Design review of the part shown in the three views and the two pictorial views. Dimensions are in mm from the part's minimum x, y and z. A direction names the side the tool comes from. Round coordinates to 2 decimals unless told otherwise and drop trailing zeros. Loops run counter-clockwise (first coordinate to the right, second up) from the corner with the lowest first, then second, coordinate; pieces in that order, holes last.
1. To check wall thickness, follow line 1 along Y through (x, z) = (2.6, 7); line 2 along Z through (x, y) = (3.45, 1.5); line 3 along Z through (x, y) = (2.35, 2.5). State the ranges of each line that lie inside material, in increasing order.
2. Tool access review of the marked faces 1 and 2: name each direction out of +Z, -Z, +X, -X, +Y, -Y from which nothing blocks a thin tool from reaching the whole face with its end or side.
3. Clearance check with a flat-ended pin moving along its axis: pin 1 Ø0.6 at (x, y) = (2, 2) entering from +Z. State where the tip first meets the part, or that it passes through.
4. Consider section A-A on z = 12. State the section outline as (x, y) points.
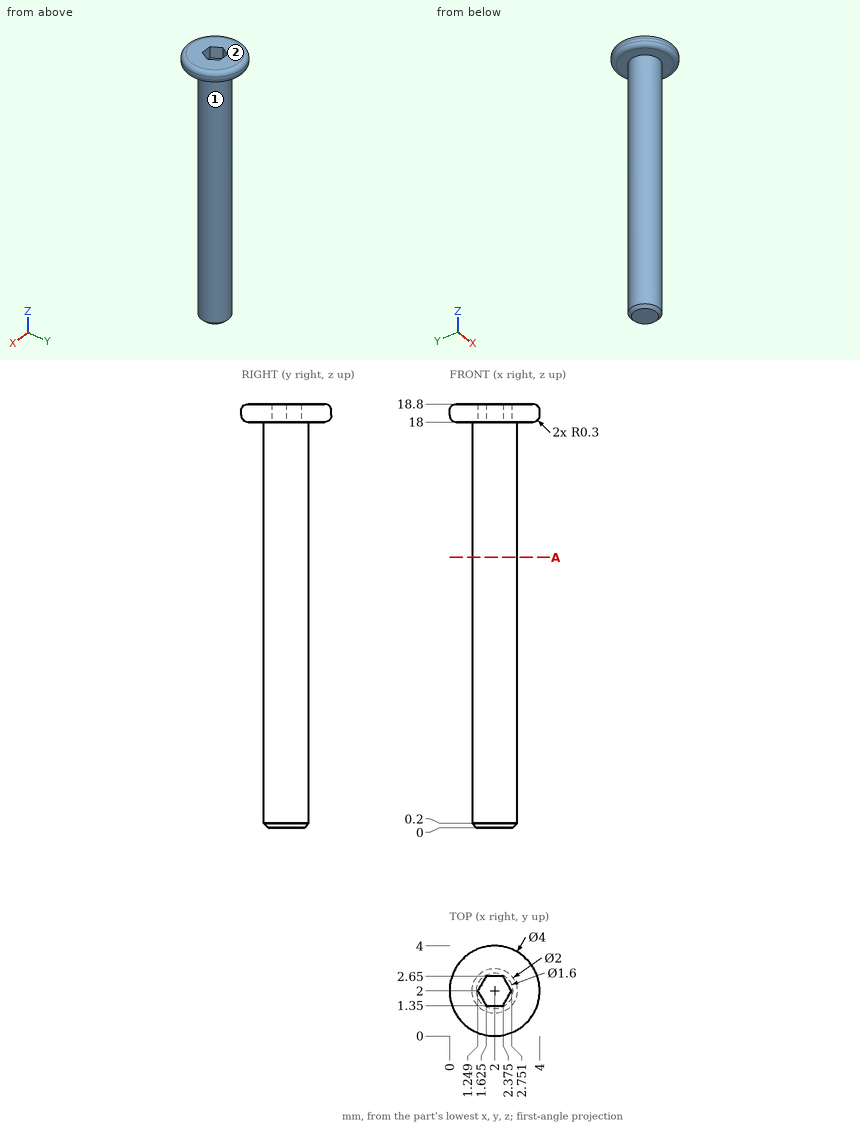
Resolved:
1. line 1: y = 1.2 to 2.8
1. line 2: z = 18 to 18.8
1. line 3: z = 0 to 18
2. face 1: -Z
2. face 2: +Z, +X, -X, +Y, -Y
3. pin 1: stops at z = 18
4. outline: circle Ø2 at (2, 2)
